Could you check a few things on this model? Use its own coordinates, in mm. Face numbers are marked on the shaded views. Coordinates: 2 decimals unless noted, no trailing zeros. Write each loop counter-clockwise with the first axis right and the second up, starting at its lowest first coordinate (ties: lowest second). Pieces come first, ordered by that corner, then holes. Notation, with made-up numbers: (45.25, 6.25) - (98.25, 6.25) arc R29 ccw to (98.25, 44.25) - close; hole circle Ø5 at (32.25, 28). An arc over 180 degrees is marked (long way). Write item = value, one per line. Start each with the question number.
```python
from build123d import *

# Parameters (mm, degrees)
SKETCH1_W                            = 78
SKETCH1_H                            = 70
BOSS_EXTRUDE1_DEPTH                  = 12
F_17_0_17_DIAMETER_HOLE1_D           = 17
F_17_0_17_DIAMETER_HOLE1_DEPTH       = 25
F_17_0_17_DIAMETER_HOLE1_CSINK_D     = 17.05
F_17_0_17_DIAMETER_HOLE1_CSINK_ANGLE = 90
F_17_0_17_DIAMETER_HOLE1_TIP         = 5.107315262
F_3_0_3_DIAMETER_HOLE2_D             = 3
F_3_0_3_DIAMETER_HOLE2_CSINK_D       = 3.05
F_3_0_3_DIAMETER_HOLE2_CSINK_ANGLE   = 90
CUT_EXTRUDE1_REACH                   = 83.025
SKETCH11_R                           = 14
CUT_EXTRUDE2_REACH                   = 59.637


with BuildPart() as part:
    # Sketch1 → Boss-Extrude1 (new, symmetric)
    with BuildSketch(Plane.XY):
        Rectangle(SKETCH1_W, SKETCH1_H)
    extrude(amount=BOSS_EXTRUDE1_DEPTH, both=True)

    # Ø17.0 (17) Diameter Hole1
    with Locations(Plane(origin=(0, 35, 0), x_dir=(1, 0, 0), z_dir=(0, 1, 0))):
        with Locations((0, 0)):
            CounterSinkHole(F_17_0_17_DIAMETER_HOLE1_D / 2, F_17_0_17_DIAMETER_HOLE1_CSINK_D / 2, depth=F_17_0_17_DIAMETER_HOLE1_DEPTH, counter_sink_angle=F_17_0_17_DIAMETER_HOLE1_CSINK_ANGLE)
            with Locations((0, 0, -(F_17_0_17_DIAMETER_HOLE1_DEPTH + F_17_0_17_DIAMETER_HOLE1_TIP / 2))):  # 118° drill point
                Cone(0, F_17_0_17_DIAMETER_HOLE1_D / 2, F_17_0_17_DIAMETER_HOLE1_TIP, mode=Mode.SUBTRACT)

    # Ø3.0 (3) Diameter Hole2 (through all)
    with Locations(Plane.XY.offset(12)):
        with Locations((8.5, 23)):
            CounterSinkHole(F_3_0_3_DIAMETER_HOLE2_D / 2, F_3_0_3_DIAMETER_HOLE2_CSINK_D / 2, counter_sink_angle=F_3_0_3_DIAMETER_HOLE2_CSINK_ANGLE)

    # Sketch11 → Cut-Extrude1 (cut, up to next)
    with BuildSketch(Plane(origin=(0, 35, 0), x_dir=(1, 0, 0), z_dir=(0, 1, 0)), mode=Mode.PRIVATE) as cut_extrude1_sk1:
        with Locations((-47.8, 0)):
            Circle(SKETCH11_R)
    cut_extrude1_tool1 = extrude(cut_extrude1_sk1.sketch, amount=-CUT_EXTRUDE1_REACH, mode=Mode.PRIVATE) & part.part
    # Sketch11 → Cut-Extrude1 (cut, up to next)
    with BuildSketch(Plane(origin=(0, 35, 0), x_dir=(1, 0, 0), z_dir=(0, 1, 0)), mode=Mode.PRIVATE) as cut_extrude1_sk2:
        with Locations((47.8, 0)):
            Circle(SKETCH11_R)
    cut_extrude1_tool2 = extrude(cut_extrude1_sk2.sketch, amount=-CUT_EXTRUDE1_REACH, mode=Mode.PRIVATE) & part.part
    add(cut_extrude1_tool1.solids().sort_by_distance((-47.8, 35, 0))[0], mode=Mode.SUBTRACT)
    add(cut_extrude1_tool2.solids().sort_by_distance((47.8, 35, 0))[0], mode=Mode.SUBTRACT)

    # Sketch12 → Cut-Extrude2 (cut, up to next)
    with BuildSketch(Plane.XY.offset(12), mode=Mode.PRIVATE) as cut_extrude2_sk1:
        Polygon((27, -35), (27, -32), (24, -32), (24, -29), (21, -29), (21, -26), (18, -26), (18, -23), (15, -23), (15, -20), (12, -20), (12, -17), (9, -17), (9, -14), (6, -14), (6, -11), (3, -11), (3, -8), (-3, -8), (-3, -11), (-6, -11), (-6, -14), (-9, -14), (-9, -17), (-12, -17), (-12, -20), (-15, -20), (-15, -23), (-18, -23), (-18, -26), (-21, -26), (-21, -29), (-24, -29), (-24, -32), (-27, -32), (-27, -35), align=None)
    cut_extrude2_tool1 = extrude(cut_extrude2_sk1.sketch, amount=-CUT_EXTRUDE2_REACH, mode=Mode.PRIVATE) & part.part
    add(cut_extrude2_tool1.solids().sort_by_distance((0, -25.5, 12))[0], mode=Mode.SUBTRACT)


solid = part.part
```
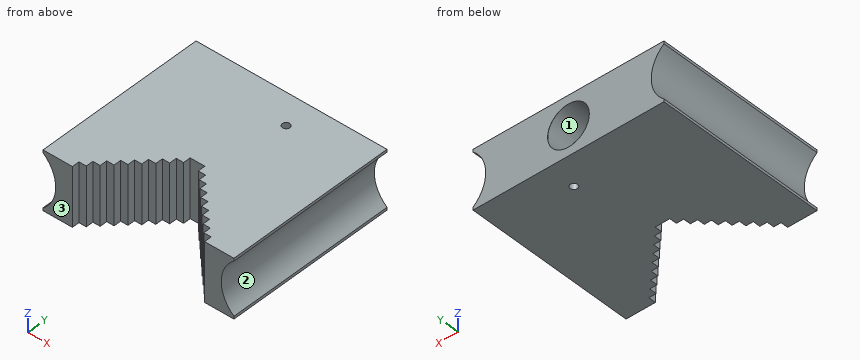
1) If I drill on probe 1 along Y at (x, z) = (8.5, 4.25); probe 2 along Z at (x, y) = (0, 25); probe 3 along X at (y, z) = (23, 0.25), over which ranges is the centre line in solid material (lowest first)? Write a range as [from, to].
2) Suppose I cut it at A-A on y = -30. Please give me the cut outline in (x, z).
3) Suppose I cut it at B-B on y = 20.5. Please give me the cut outline in (x, z), plus the area to 3 significant figures.
4) Thinking about a two-plate mould opening in X: for the marked faces 1, 2 and 3, which applies, +X half, -X half, draft (parallel to the pull), parting line (faces both ways), or undercut?
5) Suppose I cut it at C-C on x = 25.5. Please give me the cut outline in (y, z).
6) For P1, Ø0.9, axis at x = 10, z = 3, coming from the -Y side; P2, Ø13.5, axis at x = 0, z = 0, coming from the +Y side; P3, Ø12, axis at y = 20, z = -1.5, coming from the -X side, each with a flat end and sliding along its axis, tell me the tip position at first contact or that it passes through.
Reply:
q1.probe_1 = [-14, 21.5], [24.5, 35]
q1.probe_2 = [-12, -8.5], [8.5, 12]
q1.probe_3 = [-33.8, -8.5], [10, 33.8]
q2.outline = (-39, -12) - (-24, -12) - (-24, 12) - (-39, 12) - (-39, 10.89) arc R14 cw to (-39, -10.89) - close; (24, -12) - (39, -12) - (39, -10.89) arc R14 cw to (39, 10.89) - (39, 12) - (24, 12) - close
q3.outline = (-39, -12) - (39, -12) - (39, -10.89) arc R14 cw to (39, 10.89) - (39, 12) - (-39, 12) - (-39, 10.89) arc R14 cw to (-39, -10.89) - close; hole circle Ø17 at (0, 0)
q3.area = 1,490 mm^2
q4.face_1 = undercut
q4.face_2 = +X half
q4.face_3 = draft
q5.outline = (-32, -12) - (35, -12) - (35, 12) - (-32, 12) - close
q6.P1 = -17
q6.P2 = 8.95
q6.P3 = -35.98
